Geometry: final body of the model. Coordinates: model frame, mm. A direction names the side the tool comes from. Coordinates: 2 decimals unless noted, no trailing zeros. Order: outer loops, then holes, each group sorted by start corner. A loop starts at its lowest first (then second) coordinate and runs counter-clockwise, first axis right, second up. Notation, with made-up numbers: (78.25, 19.25) - (115.25, 19.25) arc R22 cw to (115.25, 30.25) - close; hole circle Ø2 at (45.5, -4.5). An arc over 180 degrees is marked (long way). Use a Markdown table: item, result. Add a question column.
```python
from build123d import *

# Parameters (mm, degrees)
F0_W        = 38.1
F0_H        = 101.6
F1_DEPTH    = 30.48
F2_T1_DEPTH = 157.48
F5_DEPTH    = 5.08
F6_T1_DEPTH = 114.3
F6_T4_ANGLE = 161.4904654603
F6_T6_ANGLE = 161.4904654612


# Not quite as in the source:
# - a fillet or chamfer that OpenCascade refuses, or shapes differently, is made with other operations: its cross-section is extruded or revolved along the edge and cut away or added


with BuildPart() as f1:
    # F0 (on Top) → F1 (new body)
    with BuildSketch(Plane.XY):
        with Locations((-7.3909840986, -8.8067197621)):
            Rectangle(F0_W, F0_H)
    extrude(amount=F1_DEPTH)

    # F2: fillet of radius 25.4 on 2 edges, made by hand

    # F2_s2 → F2_t1 (cut)
    with BuildSketch(Plane.XY.offset(-63.5)):
        with BuildLine():
            ThreePointArc((-13.7409840986, -59.6067197621), (4.2195281435, -52.1672320042), (11.6590159014, -34.2067197621))
            Line((11.6590159014, -34.2067197621), (11.6590159014, -59.6067197621))
            Line((11.6590159014, -59.6067197621), (-13.7409840986, -59.6067197621))
        make_face()
        with BuildLine():
            ThreePointArc((-26.4409840986, -34.2067197621), (-19.0014963408, -52.1672320042), (-1.0409840986, -59.6067197621))
            Line((-1.0409840986, -59.6067197621), (-26.4409840986, -59.6067197621))
            Line((-26.4409840986, -59.6067197621), (-26.4409840986, -34.2067197621))
        make_face()
    extrude(amount=F2_T1_DEPTH, mode=Mode.SUBTRACT)

    # F4 (on offset) → F5 (join)
    with BuildSketch(Plane.YZ.offset(-5.08)):
        with BuildLine():
            Line((-14.0174488836, -16.263814643), (-11.133858472, -16.263814643))
            ThreePointArc((-11.133858472, -16.263814643), (-2.2681486848, -0.0339935381), (11.991857098, -11.8093974888))
            ThreePointArc((11.991857098, -11.8093974888), (11.7754039507, -14.0775461736), (11.133858472, -16.263814643))
            Line((11.133858472, -16.263814643), (14.0174488836, -16.263814643))
            ThreePointArc((14.0174488836, -16.263814643), (14.5344751626, -14.0632247081), (14.7081849794, -11.8093974888))
            ThreePointArc((14.7081849794, -11.8093974888), (-2.2538272193, 2.7250776738), (-14.0174488836, -16.263814643))
        make_face()
        with BuildLine():
            ThreePointArc((-10.936740827, -17.3538234085), (-10.9902716166, -16.8006761373), (-11.133858472, -16.263814643))
            Line((-11.133858472, -16.263814643), (-14.0174488836, -16.263814643))
            ThreePointArc((-14.0174488836, -16.263814643), (-14.0054514358, -16.2990621553), (-13.9947204643, -16.3347156561))
            ThreePointArc((-13.9947204643, -16.3347156561), (-13.8183302749, -16.8476961899), (-13.6231437858, -17.3538234085))
            Line((-13.6231437858, -17.3538234085), (-10.936740827, -17.3538234085))
        make_face()
        with BuildLine():
            Line((14.0174488836, -16.263814643), (11.133858472, -16.263814643))
            ThreePointArc((11.133858472, -16.263814643), (10.9810910084, -16.799907635), (10.9185537399, -17.3538234085))
            Line((10.9185537399, -17.3538234085), (13.6231437858, -17.3538234085))
            ThreePointArc((13.6231437858, -17.3538234085), (13.781697315, -16.9470549808), (13.9281083774, -16.5357599818))
            ThreePointArc((13.9281083774, -16.5357599818), (13.9637636905, -16.3968256904), (14.0174488836, -16.263814643))
        make_face()
        with BuildLine():
            ThreePointArc((-11.1015096713, -18.4438321739), (-10.9743154761, -17.9056013647), (-10.936740827, -17.3538234085))
            Line((-10.936740827, -17.3538234085), (-13.6231437858, -17.3538234085))
            ThreePointArc((-13.6231437858, -17.3538234085), (-13.3861112566, -17.9038811268), (-13.1268801243, -18.4438321739))
            Line((-13.1268801243, -18.4438321739), (-11.1015096713, -18.4438321739))
        make_face()
        with BuildLine():
            Line((13.6231437858, -17.3538234085), (10.9185537399, -17.3538234085))
            ThreePointArc((10.9185537399, -17.3538234085), (10.9471844464, -17.9048318245), (11.0651192382, -18.4438321739))
            Line((11.0651192382, -18.4438321739), (13.1268801243, -18.4438321739))
            ThreePointArc((13.1268801243, -18.4438321739), (13.3861112566, -17.9038811268), (13.6231437858, -17.3538234085))
        make_face()
        with BuildLine():
            ThreePointArc((-13.6231437858, -17.3538234085), (-13.8183302749, -16.8476961899), (-13.9947204643, -16.3347156561))
            ThreePointArc((-13.9947204643, -16.3347156561), (-13.9894299583, -16.8803028031), (-14.2604863377, -17.3538234085))
            Line((-14.2604863377, -17.3538234085), (-13.6231437858, -17.3538234085))
        make_face()
        with BuildLine():
            ThreePointArc((-13.1268801243, -18.4438321739), (-13.3861112566, -17.9038811268), (-13.6231437858, -17.3538234085))
            Line((-13.6231437858, -17.3538234085), (-14.2604863377, -17.3538234085))
            ThreePointArc((-14.2604863377, -17.3538234085), (-14.9980791155, -17.659647367), (-15.7356718933, -17.3538234085))
            Line((-15.7356718933, -17.3538234085), (-16.868545512, -17.3538234085))
            ThreePointArc((-16.868545512, -17.3538234085), (-17.3451536393, -17.8087510018), (-17.5206139684, -18.4438321739))
            Line((-17.5206139684, -18.4438321739), (-13.1268801243, -18.4438321739))
        make_face()
        with BuildLine():
            ThreePointArc((-12.195911288, -20.0307388176), (-11.5329900367, -19.3170914758), (-11.1015096713, -18.4438321739))
            Line((-11.1015096713, -18.4438321739), (-13.1268801243, -18.4438321739))
            ThreePointArc((-13.1268801243, -18.4438321739), (-12.6862330658, -19.2518564902), (-12.195911288, -20.0307388176))
        make_face()
        with BuildLine():
            ThreePointArc((14.1034464611, -17.3538234085), (13.9336822531, -16.962387408), (13.9281083774, -16.5357599818))
            ThreePointArc((13.9281083774, -16.5357599818), (13.781697315, -16.9470549808), (13.6231437858, -17.3538234085))
            Line((13.6231437858, -17.3538234085), (14.1034464611, -17.3538234085))
        make_face()
        with BuildLine():
            Line((14.1034464611, -17.3538234085), (13.6231437858, -17.3538234085))
            ThreePointArc((13.6231437858, -17.3538234085), (13.3861112566, -17.9038811268), (13.1268801243, -18.4438321739))
            Line((13.1268801243, -18.4438321739), (17.526, -18.4438321739))
            Line((17.526, -18.4438321739), (17.526, -17.8258201323))
            ThreePointArc((17.526, -17.8258201323), (17.4025849977, -17.5677526977), (17.2126789083, -17.3538234085))
            Line((17.2126789083, -17.3538234085), (15.8839765936, -17.3538234085))
            ThreePointArc((15.8839765936, -17.3538234085), (14.9937115274, -17.8192920932), (14.1034464611, -17.3538234085))
        make_face()
        with BuildLine():
            Line((13.1268801243, -18.4438321739), (11.0651192382, -18.4438321739))
            ThreePointArc((11.0651192382, -18.4438321739), (11.4934563351, -19.3420700335), (12.1649032036, -20.0765514995))
            ThreePointArc((12.1649032036, -20.0765514995), (12.6722144503, -19.2757008789), (13.1268801243, -18.4438321739))
        make_face()
        with BuildLine():
            ThreePointArc((-12.195911288, -20.0307388176), (-12.6862330658, -19.2518564902), (-13.1268801243, -18.4438321739))
            Line((-13.1268801243, -18.4438321739), (-17.5206139684, -18.4438321739))
            ThreePointArc((-17.5206139684, -18.4438321739), (-15.2749066717, -20.6352919031), (-12.195911288, -20.0307388176))
        make_face()
        with BuildLine():
            Line((17.526, -18.4438321739), (13.1268801243, -18.4438321739))
            ThreePointArc((13.1268801243, -18.4438321739), (12.6722144503, -19.2757008789), (12.1649032036, -20.0765514995))
            ThreePointArc((12.1649032036, -20.0765514995), (15.2798483428, -20.6865502684), (17.526, -18.4438321739))
        make_face()
        with BuildLine():
            Line((-16.868545512, -17.3538234085), (-15.7356718933, -17.3538234085))
            ThreePointArc((-15.7356718933, -17.3538234085), (-15.7525545617, -17.3365203222), (-15.769031426, -17.3188303749))
            ThreePointArc((-15.769031426, -17.3188303749), (-16.3228921506, -17.2073853467), (-16.868545512, -17.3538234085))
        make_face()
        with BuildLine():
            ThreePointArc((17.2126789083, -17.3538234085), (16.548327751, -17.1094834068), (15.8839765936, -17.3538234085))
            Line((15.8839765936, -17.3538234085), (17.2126789083, -17.3538234085))
        make_face()
        with BuildLine():
            ThreePointArc((17.526, -18.4438321739), (17.5736704973, -18.1348261531), (17.526, -17.8258201323))
            Line((17.526, -17.8258201323), (17.526, -18.4438321739))
        make_face()
    extrude(amount=-F5_DEPTH)

    # F6: fillet of radius 15.24 on 4 edges, made by hand

    # F6_s2 → F6_t1 (cut)
    with BuildSketch(Plane.XZ.offset(-80.0932802379)):
        with BuildLine():
            ThreePointArc((11.6590159014, 15.24), (7.1953232467, 4.4636926547), (-3.5809840986, 0))
            Line((-3.5809840986, 0), (11.6590159014, 0))
            Line((11.6590159014, 0), (11.6590159014, 15.24))
        make_face()
        with BuildLine():
            ThreePointArc((-26.4409840986, 15.24), (-21.9772914439, 4.4636926547), (-11.2009840986, 0))
            Line((-11.2009840986, 0), (-26.4409840986, 0))
            Line((-26.4409840986, 0), (-26.4409840986, 15.24))
        make_face()
    extrude(amount=F6_T1_DEPTH, mode=Mode.SUBTRACT)

    # F6_s3 → F6_t4 (revolve, cut)
    with BuildSketch(Plane.XZ.offset(34.206719762)):
        with BuildLine():
            ThreePointArc((-3.5809840986, 0), (7.1953232467, 4.4636926547), (11.6590159014, 15.24))
            Line((11.6590159014, 15.24), (11.6590159014, 0))
            Line((11.6590159014, 0), (-3.5809840986, 0))
        make_face()
    revolve(axis=Axis((-13.7409840987, -34.206719762, 0), (0, 0, -1)), revolution_arc=F6_T4_ANGLE, mode=Mode.SUBTRACT)

    # F6_s5 → F6_t6 (revolve, cut)
    with BuildSketch(Plane(origin=(-10.402517324, -31.0726622139, 0), x_dir=(0, 0, 1), z_dir=(0.3174624617, 0.9482708397, 0))):
        with BuildLine():
            ThreePointArc((0, 20.0322145968), (4.4636926547, 30.8085219421), (15.24, 35.2722145968))
            Line((15.24, 35.2722145968), (0, 35.2722145968))
            Line((0, 35.2722145968), (0, 20.0322145968))
        make_face()
    revolve(axis=Axis((-1.0409840986, -34.2067197621, 0), (0, 0, -1)), revolution_arc=F6_T6_ANGLE, mode=Mode.SUBTRACT)


solid = f1.part
```
1) First-contact query: pin 1 (12.5 mm diameter, centred on y = 10.5, z = -12.5, fed in from +X); pin 2 (6 mm diameter, centred on y = -2.5, z = 4, fed in from +X); pin 3 (17 mm diameter, centred on y = 12, z = -12, fed in from -X); pin 4 (1 mm diameter, centred on x = 3, z = -0.5, fed in from -Y). Flat tips, straight axial feed; report the tip coordinate or a pass-through.
2) Draft query along Y for faces 1 (the flat face through (-8, 41.993, 15)), 2 (the cylindrical face through (-7.58, -10.55, -6.11)), 3 (the cylindrical face through (7.31, 4.43, 4.58)). Return one class per face: released by +Y, released by -Y, zero draft, split by the parting line, or undercut.
3) Section query A-A (z = -2.5). Return the cut outline in (x, y), and give its area (3 significant figures).
4) Line query: line 1 (Z direction, x = -11.5, y = 25); line 2 (X direction, y = 32, z = 15); line 3 (Z direction, x = 7.5, y = -25.5). Output: solid intervals per line, ascending. Write a range as from..to.
5) Section query B-B (y = 36). Return the cut outline in (x, z), and give its area (3 significant figures).
6) Access query for faces 4 (the flat face through (-5.08, -12.13, -11.11)), 5 (the cylindrical face through (6.195, -49.946, 22.753)), 6 (the flat face through (-10.16, -12.13, -11.11)). Directions: +Z, -Z, +X, -X, +Y, -Y. A direction counts if a zero-diameter tool reaches every point of the face in a straight line with its end or side. Return the directions, or none.
From the geometry:
| question | item | result |
|---|---|---|
| 1 | pin 1 | stops at x = -5.08 |
| 1 | pin 2 | stops at x = 9.24 |
| 1 | pin 3 | stops at x = -10.16 |
| 1 | pin 4 | passes through |
| 2 | face 1 | released by +Y |
| 2 | face 2 | undercut |
| 2 | face 3 | zero draft |
| 3 | outline | (-10.16, -11.39) - (-5.08, -11.39) - (-5.08, -7.56) - (-10.16, -7.56) - close; (-10.16, 7.56) - (-5.08, 7.56) - (-5.08, 11.39) - (-10.16, 11.39) - close |
| 3 | area | 38.9 mm^2 |
| 4 | line 1 | z = 0..30.48 |
| 4 | line 2 | x = -26.44..11.66 |
| 4 | line 3 | z = 4.78..30.48 |
| 5 | outline | (-26.44, 15.24) arc R15.24 ccw to (-11.2, 0) - (-3.58, 0) arc R15.24 ccw to (11.66, 15.24) - (11.66, 30.48) - (-26.44, 30.48) - close |
| 5 | area | 1,060 mm^2 |
| 6 | face 4 | -Z, +X, +Y, -Y |
| 6 | face 5 | +Z, -Z, +X, -Y |
| 6 | face 6 | -Z, -X, +Y, -Y |
